Autodesk Inventor part; units mm, degrees
ref_plane "YZ Plane" through (0, 0, 0) normal (1, 0, 0) x (0, 1, 0)
ref_plane "XZ Plane" through (0, 0, 0) normal (0, 1, 0) x (-1, 0, 0)
ref_plane "XY Plane" through (0, 0, 0) normal (0, 0, 1) x (1, 0, 0)
sketch "Sketch1" plane through (0, 0, 0) normal (0, 0, 1) x (1, 0, 0)
  line L0 (-3.7865, -1.449) -> (13.2135, -1.449)
  line L1 (13.2135, -1.449) -> (13.2135, -2.949)
  line L2 (13.2135, -2.949) -> (-3.7865, -2.949)
  line L3 (-3.7865, -2.949) -> (-3.7865, -1.449)
  line L4 (-3.7865, -2.949) -> (-2.2865, -2.949)
  line L5 (-3.7865, -12.949) -> (-3.7865, -2.949)
  line L6 (3.2135, -16.449) -> (3.2135, -17.949)
  line L7 (3.2135, -17.949) -> (1.2135, -17.949)
  arc A0 (3.2135, -16.449) -> (7.7135, -11.949) centre (2.4495, -11.1849) ccw
  line L8 (7.7135, -11.949) -> (9.2135, -11.949)
  arc A1 (3.2135, -17.949) -> (9.2135, -11.949) centre (3.2135, -11.949) ccw
  arc A2 (-3.7865, -12.949) -> (1.2135, -17.949) centre (1.2135, -12.949) ccw
  arc A3 (-2.2865, -12.949) -> (1.2135, -16.449) centre (1.2135, -12.949) ccw
  line L9 (-3.7865, -12.949) -> (-2.2865, -12.949)
  line L10 (1.2135, -17.949) -> (1.2135, -16.449)
  line L11 (1.2135, -16.449) -> (3.2135, -16.449)
  line L12 (-2.2865, -2.949) -> (-2.2865, -12.949)
  point P0 (0, 0)
  dimension "d0" = 1.5
  dimension "d2" = 1.5
  dimension "d3" = 6
  dimension "d4" = 5
  dimension "d5" = 5
  dimension "d7" = 6
  dimension "d8" = 2
  dimension "d12" = 15.5
  dimension "d13" = 10
  dimension "d23" = 1.5
extrude "Extrusion1" add sketch "Sketch1" along normal blind 50
sketch "Sketch2" plane through (-2.2865, -2.949, 0) normal (0, -1, 0) x (1, 0, 0)
  line L0 (15.5, 50) -> (-1.5, 50)
  line L1 (10.5, 50) -> (10.5, 0) construction
  line L2 (15.5, 0) -> (-1.5, 0)
  line L3 (15.5, 0) -> (-1.5, 0)
  line L4 (-1.5, 0) -> (-1.5, 50)
  line L5 (15.5, 50) -> (-1.5, 50)
  line L6 (15.5, 0) -> (15.5, 50)
  circle A0 centre (10.5, 44.75) radius 2.25
  circle A1 centre (10.5, 5.25) radius 2.25
  point P0 (2.2865, 0)
  dimension "d14" = 5
  dimension "d15" = 4.5
  dimension "d16" = 4.5
  dimension "d18" = 3
  dimension "d19" = 3
extrude "Extrusion2" cut sketch "Sketch2" against normal blind 3 contours A0 | A1
properties part number "TopHook"
Could you check a few things on this model? Use its own coordinates, in mm. A direction names the side the tool comes from. Give positions to 0.01 mm unless a question says otherwise; leave off trailing zeros. Write each loop counter-clockwise with the first axis right and the second up, starting at its lowest first coordinate (ties: lowest second). Pieces come first, ordered by that corner, then holes. Notation, with made-up numbers: (57.25, 62.5) -> (104.25, 62.5) arc R9 ccw to (104.25, 71.5) -> close; hole circle Ø10 at (4, 34.25). An arc over 180 degrees is marked (long way). Answer as a JSON object with one key per item and string values.
Q1. We'd pull the mould along Y, two halves only. Please class faces 6 (the flat face through (5, -1.449, 25)), 7 (the flat face through (2, -16.449, 25)), 8 (the flat face through (-3, -8, 0)), 9 (the cylindrical face through (-2.283, -16.523, 24.65)): released by +Y, released by -Y, zero draft, split by the parting line, or undercut.
Taken from the geometry:
{"face 6": "released by +Y", "face 7": "undercut", "face 8": "zero draft", "face 9": "released by -Y"}
Q2. Suppose I cut it at A-A on z = 5.25. Write out the boundary of the cut face in (x, y), then the cut area to 3 significant figures.
Taken from the geometry:
{"outline": "(-3.79, -12.95) arc R5 ccw to (1.21, -17.95) -> (3.21, -17.95) arc R6 ccw to (9.21, -11.95) -> (7.71, -11.95) arc R5.32 cw to (3.21, -16.45) -> (1.21, -16.45) arc R3.5 cw to (-2.29, -12.95) -> (-2.29, -2.95) -> (5.96, -2.95) -> (5.96, -1.45) -> (-3.79, -1.45) -> close; (10.46, -2.95) -> (13.21, -2.95) -> (13.21, -1.45) -> (10.46, -1.45) -> close", "area": "60.3 mm²"}
Q3. Suppose I cut it at B-B on y = -4.5. Write out the boundary of the cut face in (x, z).
Taken from the geometry:
{"outline": "(-3.79, 0) -> (-2.29, 0) -> (-2.29, 50) -> (-3.79, 50) -> close"}
Q4. Which directions (+Z, -Z, +X, -X, +Y, -Y) give clear straight access to the entire face, cutting with the end or side of a thin tool? Please do faces 1 (the cylindrical face through (7.503, -16.145, 24.65)), 2 (the cylindrical face through (6.244, -14.912, 24.65)), 3 (the flat face through (2, -17.949, 25)), 4 (the cylindrical face through (7.92, -2.21, 46.98)), 5 (the flat face through (6, -2.949, 25)).
Taken from the geometry:
{"face 1": "+Z, -Z, +X, -Y", "face 2": "+Z, -Z", "face 3": "+Z, -Z, +X, -X, -Y", "face 4": "+Y", "face 5": "+Z, -Z, +X"}
Q5. Suppose I cut it at D-D on z = 44. Write out the boundary of the cut face in (x, y), then the cut area to 3 significant figures.
Taken from the geometry:
{"outline": "(-3.79, -12.95) arc R5 ccw to (1.21, -17.95) -> (3.21, -17.95) arc R6 ccw to (9.21, -11.95) -> (7.71, -11.95) arc R5.32 cw to (3.21, -16.45) -> (1.21, -16.45) arc R3.5 cw to (-2.29, -12.95) -> (-2.29, -2.95) -> (6.09, -2.95) -> (6.09, -1.45) -> (-3.79, -1.45) -> close; (10.33, -2.95) -> (13.21, -2.95) -> (13.21, -1.45) -> (10.33, -1.45) -> close", "area": "60.7 mm²"}
Q6. Please list where these lines run through material, in increasing order: L1, parallel to Z at x = 8.75, y = -2.75; L2, parallel to Y at x = 10.75, z = 22; L3, parallel to Y at x = 0.75, z = 2.
Taken from the geometry:
{"L1": "z = 0 to 3.06, 7.44 to 42.56, 46.94 to 50", "L2": "y = -2.95 to -1.45", "L3": "y = -17.93 to -16.42, -2.95 to -1.45"}
Q7. Will these pins go through, and if not, where does the flat tip stop? pin 1 Ø5 at (x, y) = (5, -12) entering from -Z; pin 2 Ø5 at (x, z) = (8.21, 5.25) entering from -Y; pin 3 Ø3.5 at (x, z) = (8.21, 44.75) entering from -Y.
Taken from the geometry:
{"pin 1": "passes through", "pin 2": "stops at y = -17.4", "pin 3": "stops at y = -16.99"}
Q8. Suppose I cut it at C-C on x = 12.25. Write out the boundary of the cut face in (y, z), then the cut area to 3 significant figures.
Taken from the geometry:
{"outline": "(-2.95, 0) -> (-1.45, 0) -> (-1.45, 50) -> (-2.95, 50) -> close", "area": "75.0 mm²"}
